```python
from build123d import *

# Parameters (mm, degrees)
F1_DEPTH = 580
F3_D     = 11
F4_SIZE  = 5


with BuildPart() as f1:
    # F0 (on Front) → F1 (new body)
    with BuildSketch(Plane.XZ):
        Polygon((28, 0), (0, 0), (0, -15), (8, -15), (8, -31), (0, -31), (0, -52.9289321881), (7.0710678119, -60), (28, -60), align=None)
    extrude(amount=F1_DEPTH)

    # F3 (through all)
    with Locations(Plane.YZ.offset(28)):
        with Locations((-555, -23), (-422.5, -23), (-290, -23), (-157.5, -23), (-25, -23)):
            Hole(F3_D / 2)

    # F4
    f4_edges = [f1.edges().sort_by_distance(p)[0] for p in [
        (28, -290, -60),
    ]]
    chamfer(f4_edges, length=F4_SIZE)


solid = f1.part
```
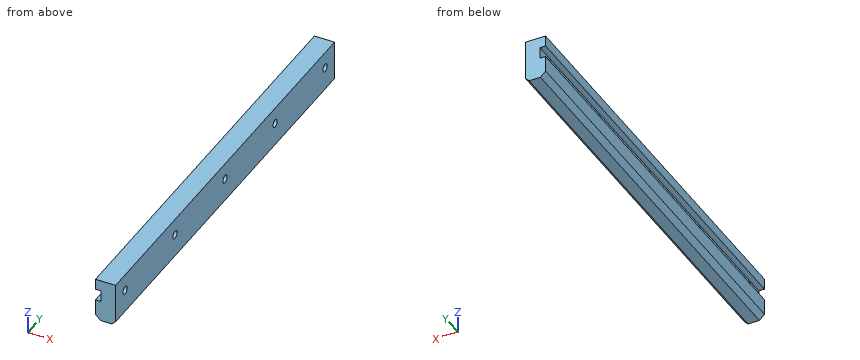
Geometry: final body of the model. Coordinates: model frame, mm. Round coordinates to 2 decimals unless told otherwise and drop trailing zeros. Order: outer loops, then holes, each group sorted by start corner. A loop starts at its lowest first (then second) coordinate and runs counter-clockwise, first axis right, second up. Notation, with made-up numbers: (28.25, 43.5) -> (77.25, 43.5) arc R14 cw to (77.25, 48.5) -> close; hole circle Ø7 at (28.25, 68.25). An arc over 180 degrees is marked (long way). Use CSV: the item, a comma, the result in double quotes. Start each with the question number.
1) Section C-C (y = -183.5). Return the cut outline in (x, z).
2) First-contact query: pin 1 Ø9 at (x, y) = (3, -402) entering from -Z; pin 2 Ø6.5 at (y, z) = (-422.5, -23) entering from +X; pin 3 Ø8 at (y, z) = (-247.5, -23) entering from -X. Flat tips, straight axial feed; report the tip coordinate or a pass-through.
3) Section A-A (z = -23). Return the cut outline in (x, y).
4) Section B-B (y = -25). Return the cut outline in (x, z).
5) Material intervals for line 1 along Z through (x, y) = (16.25, -555); line 2 along Z through (x, y) = (2, -540.5); line 3 along X through (y, z) = (-128, -53), sorted ascending. Write a range as from..to.
Returned:
1,outline,"(0, -52.93) -> (7.07, -60) -> (23, -60) -> (28, -55) -> (28, 0) -> (0, 0) -> (0, -15) -> (8, -15) -> (8, -31) -> (0, -31) -> close"
2,pin 1,"stops at z = -60"
2,pin 2,"passes through"
2,pin 3,"stops at x = 8"
3,outline,"(8, -580) -> (28, -580) -> (28, -560.5) -> (8, -560.5) -> close; (8, -549.5) -> (28, -549.5) -> (28, -428) -> (8, -428) -> close; (8, -417) -> (28, -417) -> (28, -295.5) -> (8, -295.5) -> close; (8, -284.5) -> (28, -284.5) -> (28, -163) -> (8, -163) -> close; (8, -152) -> (28, -152) -> (28, -30.5) -> (8, -30.5) -> close; (8, -19.5) -> (28, -19.5) -> (28, 0) -> (8, 0) -> close"
4,outline,"(0, -52.93) -> (7.07, -60) -> (23, -60) -> (28, -55) -> (28, -28.5) -> (8, -28.5) -> (8, -31) -> (0, -31) -> close; (0, -15) -> (8, -15) -> (8, -17.5) -> (28, -17.5) -> (28, 0) -> (0, 0) -> close"
5,line 1,"z = -60..-28.5, -17.5..0"
5,line 2,"z = -54.93..-31, -15..0"
5,line 3,"x = 0.07..28"
